Geometry check sheet. Reference: the model listing, model coordinates, mm. A direction names the side the tool comes from. Give positions to 0.01 mm unless a question says otherwise; leave off trailing zeros. Order: outer loops, then holes, each group sorted by start corner. A loop starts at its lowest first (then second) coordinate and runs counter-clockwise, first axis right, second up.
from build123d import *

# Parameters (mm, degrees)
PAD_DEPTH       = 6
SKETCH001_R     = 12.5
PAD001_DEPTH    = 10
SKETCH002_W     = 29.813109
SKETCH002_H     = 6
POCKET_DEPTH    = 3
SKETCH003_R     = 5
POCKET001_DEPTH = 5
PAD002_DEPTH    = 2


with BuildPart() as part:
    # Sketch → Pad (new body)
    with BuildSketch(Plane.XY):
        with BuildLine():
            ThreePointArc((30, -12.5), (42.5, 0), (30, 12.5))
            Line((30, 12.5), (0, 12.5))
            ThreePointArc((0, 12.5), (-12.5, 0), (0, -12.5))
            Line((30, -12.5), (0, -12.5))
        make_face()
    extrude(amount=PAD_DEPTH)

    # Sketch001 → Pad001 (new body)
    with BuildSketch(Plane.XY.offset(6)):
        Circle(SKETCH001_R)
    extrude(amount=PAD001_DEPTH)

    # Sketch002 → Pocket (cut)
    with BuildSketch(Plane.XY.offset(16)):
        with Locations((1.105551, 0)):
            Rectangle(SKETCH002_W, SKETCH002_H)
    extrude(amount=-POCKET_DEPTH, mode=Mode.SUBTRACT)

    # Sketch003 → Pocket001 (cut)
    with BuildSketch(Plane.XY.offset(13)):
        Circle(SKETCH003_R)
    extrude(amount=POCKET001_DEPTH, mode=Mode.SUBTRACT)

    # Sketch004 → Pad002 (new body)
    with BuildSketch(Plane.XY.offset(6)):
        with BuildLine():
            ThreePointArc((24, 6), (18, 0), (24, -6))
            Line((24, -6), (30, -6))
            ThreePointArc((30, -6), (36, 0), (30, 6))
            Line((24, 6), (30, 6))
        make_face()
        with BuildLine():
            ThreePointArc((30, -3), (33, 0), (30, 3))
            Line((30, 3), (24, 3))
            ThreePointArc((24, 3), (21, 0), (24, -3))
            Line((30, -3), (24, -3))
        make_face(mode=Mode.SUBTRACT)
    extrude(amount=PAD002_DEPTH)


solid = part.part
Item 1: Gauge pin test, flat ends, axial feed: pin 1 (5 mm diameter, centred on x = 28, y = 1.5, fed in from +Z); pin 2 (4 mm diameter, centred on x = -7, y = -7.5, fed in from -Z); pin 3 (3.5 mm diameter, centred on x = -9.5, z = 14.5, fed in from +Y); pin 4 (3.5 mm diameter, centred on x = 8, z = 14, fed in from +Y). Record the tip position at first contact, or that the pin passes through.
Reported:
pin 1: stops at z = 8
pin 2: stops at z = 0
pin 3: stops at y = 9.81
pin 4: stops at y = 10.83
Item 2: Sectioned sample at B-B (y = 0). Enter the section's corners in (x, z).
Reported:
outline: (-12.5, 0) - (42.5, 0) - (42.5, 6) - (36, 6) - (36, 8) - (33, 8) - (33, 6) - (21, 6) - (21, 8) - (18, 8) - (18, 6) - (12.5, 6) - (12.5, 13) - (-12.5, 13) - close
Item 3: Sectioned sample at A-A (x = 28). Enter the section's corners in (y, z).
Reported:
outline: (-12.5, 0) - (12.5, 0) - (12.5, 6) - (6, 6) - (6, 8) - (3, 8) - (3, 6) - (-3, 6) - (-3, 8) - (-6, 8) - (-6, 6) - (-12.5, 6) - close
Item 4: Sectioned sample at C-C (x = 7.5). Enter the section's corners in (y, z).
Reported:
outline: (-12.5, 0) - (12.5, 0) - (12.5, 6) - (10, 6) - (10, 16) - (3, 16) - (3, 13) - (-3, 13) - (-3, 16) - (-10, 16) - (-10, 6) - (-12.5, 6) - close
Item 5: Sectioned sample at D-D (z = 3). Enter the section's corners in (x, y), and give its area (3 significant figures).
Reported:
outline: (0, -12.5) - (30, -12.5) arc R12.5 ccw to (30, 12.5) - (0, 12.5) arc R12.5 ccw to start
area: 1,240 mm2
Item 6: Scan lines: L1, parallel to X at y = -0.25, z = 11.75; L2, parallel to Z at x = 38, y = -4; L3, parallel to Z at x = 32, y = 5.5. Record each from-to range of solid material in increasing order.
Reported:
L1: x = -12.5 to 12.5
L2: z = 0 to 6
L3: z = 0 to 8
Item 7: Set-up check for faces 1 (the flat face through (27, 6, 7)), 2 (the cylindrical face through (36, 0, 7)), 3 (the flat face through (27, -4, 8)), 4 (the cylindrical face through (18, 0, 7)), 5 (the flat face through (8, -3, 15)): record each of +Z, -Z, +X, -X, +Y, -Y from which the full face is reachable in a straight line by a thin tool's end or side.
Reported:
face 1: +Z, +X, +Y
face 2: +Z, +X
face 3: +Z, +X, +Y, -Y
face 4: +Z
face 5: +Z, +X, -X
